Geometry: final body of the model. Coordinates: model frame, mm. A direction names the side the tool comes from. Give positions to 0.01 mm unless a question says otherwise; leave off trailing zeros. Write each loop counter-clockwise with the first axis right and the second up, starting at its lowest first coordinate (ties: lowest second). Pieces come first, ordered by that corner, then holes. Notation, with made-up numbers: M -14.75,-39 L 4.25,-39 A11 cw 4.25,-32 Z; hole C -40,39.25 d1. An arc over 180 degrees is marked long. Answer as a JSON object with one key per item and string values.
from build123d import *

# Parameters (mm, degrees)
F0_W     = 18.1707702577
F0_H     = 55.8800026774
F1_DEPTH = 8
F2_R     = 4.8885197861
F3_DEPTH = 2
F4_W     = 3.7123076618
F4_H     = 15.4353883117
F5_DEPTH = 5


with BuildPart() as f1:
    # F0 (on Top) → F1 (new body)
    with BuildSketch(Plane.XY):
        with Locations((-27.7446154505, -4.6892315149)):
            Rectangle(F0_W, F0_H)
        with BuildLine():
            add(Edge.make_bspline(
                [(-36.8300005794, 23.2507698238), (-34.2214483668, 31.493687892), (-28.9456329612, 48.1650483199), (-22.1133750602, 31.6169136543), (-18.6592303216, 23.2507698238)],
                knots=[0, 0, 0, 0, 0.4944358383, 1, 1, 1, 1], degree=3))
            Line((-36.8300005794, 23.2507698238), (-18.6592303216, 23.2507698238))
        make_face()
    extrude(amount=F1_DEPTH)

    # F2 (on face) → F3 (join)
    with BuildSketch(Plane.XY.offset(8)):
        with Locations((-28.4284614027, 25.2046156675)):
            Circle(F2_R)
    extrude(amount=F3_DEPTH)

    # F4 (on face) → F5 (join)
    with BuildSketch(Plane.XY.offset(10)):
        with Locations((-28.5261552781, 32.7269257978)):
            Rectangle(F4_W, F4_H)
        with BuildLine():
            Line((-26.6700014472, 25.0092316419), (-30.382309109, 25.0092316419))
            ThreePointArc((-30.382309109, 25.0092316419), (-28.5261552781, 22.07613801), (-26.6700014472, 25.0092316419))
        make_face()
    extrude(amount=F5_DEPTH)


solid = f1.part
1) Contact query for flat-ended pins moving along their axis: P1, Ø6, axis at x = -25.5, y = -10.5, coming from the +Z side; P2, Ø1.5, axis at y = 33.5, z = 11.5, coming from the +X side; P3, Ø3, axis at x = -23.5, z = 2, coming from the +Y side (3 decimals). Output: stop coordinate, or through.
Geometry check:
{"P1": "stops at z = 8", "P2": "stops at x = -26.67", "P3": "stops at y = 36.805"}
2) Set-up query: faces 5 (the flat face through (-30.382, 33, 12)), 6 (the flat face through (-26.67, 33, 12)), 7 (the cylindrical face through (-28.584, 22.077, 12.465)). Return all of +Z, -Z, +X, -X, +Y, -Y with unobstructed straight access to the full face (end or side cutting, diameter ignored); none if empty.
Geometry check:
{"face 5": "+Z, -X, +Y", "face 6": "+Z, +X, +Y", "face 7": "+Z"}
3) Cut plane B-B on z = 14. Return loops of the section in (x, y).
Geometry check:
{"outline": "M -30.38,25.01 A2.05 ccw long -26.67,25.01 L -26.67,40.44 L -30.38,40.44 Z"}
4) Cut plane A-A on y = 12. Return loops of the section in (x, z), and give its area (3 significant figures).
Geometry check:
{"outline": "M -36.83,0 L -18.66,0 L -18.66,8 L -36.83,8 Z", "area": "145 mm2"}
5) Pull-direction query (Z, two-part tool) for faces 1 (the flat face through (-28, -32.629, 4)), 2 (the flat face through (-29, 31, 15)), 3 (the flat face through (-28, -1, 0)), 4 (the flat face through (-29, 35, 10)); classes: pulls with the +Z half, pulls with the -Z half, needs draft (parallel to the pull), parting line crosses it, or undercut.
Geometry check:
{"face 1": "needs draft", "face 2": "pulls with the +Z half", "face 3": "pulls with the -Z half", "face 4": "undercut"}
6) Line query: line 1 (Z direction, x = -31.25, y = 20); line 2 (X direction, y = 27.5, z = 13.25); line 3 (Y direction, x = -21.5, z = 4). Output: solid intervals per line, ascending. Write a range as from..to.
Geometry check:
{"line 1": "z = 0..8", "line 2": "x = -30.38..-26.67", "line 3": "y = -32.63..29.97"}
7) Cut plane C-C on z = 8.75. Return loops of the section in (x, y), and give its area (3 significant figures).
Geometry check:
{"outline": "C -28.43,25.2 d9.78", "area": "75.1 mm2"}
